The listing builds one solid part. Answer for the finished solid, in the listing's coordinates (mm). Face numbers are marked on the shaded views. A direction names the side the tool comes from. Round coordinates to 2 decimals unless told otherwise and drop trailing zeros. Write each loop counter-clockwise with the first axis right and the second up, starting at its lowest first coordinate (ties: lowest second). Pieces come first, ordered by that corner, then holes.
Item 1: A tool of negligible diameter and unlimited length cuts with its end or side. For the marked faces 1, 2 and 3, from which of +Z, -Z, +X, -X, +Y, -Y can it reach the whole face along a straight path? Write none if from no direction.
Item 2: Each of these flat-tipped pins is pushed along its axis until it touches: pin 1 (1.5 mm diameter, centred on x = 58, y = 74.5, fed in from +Z); pin 2 (2 mm diameter, centred on x = 58.5, y = 99.5, fed in from -Z); pin 3 (2 mm diameter, centred on x = 64, y = 117, fed in from +Z). Where does it stop, or does it pass through?
Item 3: Find the intervals of material crossed by probe 1 along Z at (x, y) = (20, -50.5); probe 2 along Y at (x, z) = (24.5, -1); probe 3 along Y at (x, z) = (68.5, 15.5), in increasing order.
Item 4: Find section C-C on z = 27.5. Give the vertices of the cut face in (x, y).
Item 5: Find section D-D on y = 81. Give the vertices of the cut face in (x, z), then the cut area to 3 significant figures.
Item 6: Find section A-A on z = 0. Give the vertices of the cut face in (x, y).
Item 7: Find section B-B on x = 38.1. Give the vertices of the cut face in (y, z), then the cut area to 4 significant figures.
Item 8: For a pull along Y with two mould halves and no side action, classify the marked faces 4, 5 and 6 as +Y half, -Y half, draft (parallel to the pull), parting line (faces both ways), or undercut.
```python
from build123d import *

# Parameters (mm, degrees)
F0_W     = 127
F0_H     = 76.2
F1_DEPTH = 76.2
F2_R     = 31.75
F3_DEPTH = 76.2
F4_W     = 88.9
F4_H     = 50.8
F5_DEPTH = 76.201


with BuildPart() as f1:
    # F0 (on Right) → F1 (new body)
    with BuildSketch(Plane.YZ):
        Rectangle(F0_W, F0_H)
    extrude(amount=F1_DEPTH)

    # F2 (on face) → F3 (join)
    with BuildSketch(Plane(origin=(0, 63.5, 0), x_dir=(-1, 0, 0), z_dir=(0, 1, 0))):
        with Locations((-38.1, 0)):
            Circle(F2_R)
    extrude(amount=F3_DEPTH)

    # F4 (on face) → F5 (cut, through all)
    with BuildSketch(Plane(origin=(0, 0, 0), x_dir=(0, -1, 0), z_dir=(-1, 0, 0))):
        with Locations((6.35, 0)):
            Rectangle(F4_W, F4_H)
    extrude(amount=-F5_DEPTH, mode=Mode.SUBTRACT)


solid = f1.part
```
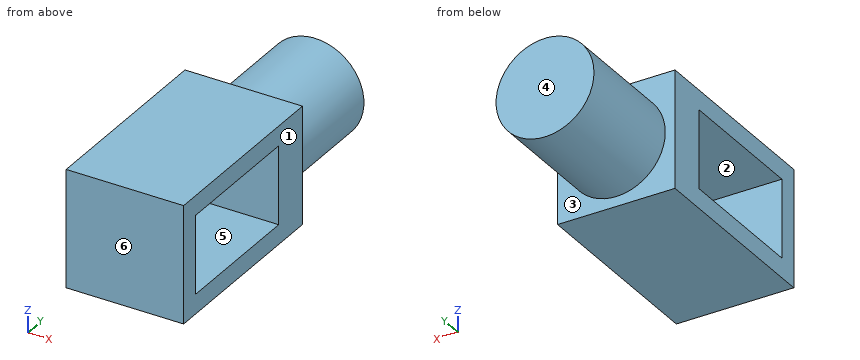
Check values:
1. face 1: +Z, -Z, +X, +Y, -Y
1. face 2: +X, -X
1. face 3: +Y
2. pin 1: stops at z = 25.32
2. pin 2: stops at z = -25.13
2. pin 3: stops at z = 19.7
3. probe 1: z = -38.1 to -25.4, 25.4 to 38.1
3. probe 2: y = -63.5 to -50.8, 38.1 to 139.7
3. probe 3: y = -63.5 to -50.8, 38.1 to 63.5
4. outline: (0, -63.5) - (76.2, -63.5) - (76.2, 63.5) - (53.97, 63.5) - (53.97, 139.7) - (22.23, 139.7) - (22.23, 63.5) - (0, 63.5) - close
5. outline: circle Ø63.5 at (38.1, 0)
5. area: 3,170 mm2
6. outline: (0, -63.5) - (76.2, -63.5) - (76.2, -50.8) - (0, -50.8) - close; (0, 38.1) - (76.2, 38.1) - (76.2, 63.5) - (69.85, 63.5) - (69.85, 139.7) - (6.35, 139.7) - (6.35, 63.5) - (0, 63.5) - close
7. outline: (-63.5, -38.1) - (63.5, -38.1) - (63.5, -31.75) - (139.7, -31.75) - (139.7, 31.75) - (63.5, 31.75) - (63.5, 38.1) - (-63.5, 38.1) - close; hole (-50.8, -25.4) - (38.1, -25.4) - (38.1, 25.4) - (-50.8, 25.4) - close
7. area: 10,000 mm2
8. face 4: +Y half
8. face 5: undercut
8. face 6: -Y half
